Read the model definition and answer for the solid it produces. Units are mm, in the model's axes. Face numbers are marked on the shaded views. Coordinates: 2 decimals unless noted, no trailing zeros. Order: outer loops, then holes, each group sorted by start corner. A loop starts at its lowest first (then second) coordinate and runs counter-clockwise, first axis right, second up. Notation, with made-up numbers: M 80.5,45.25 L 97.5,45.25 A24 ccw 97.5,74.25 Z; hole C 80.25,78 d6. An arc over 180 degrees is marked long. One line per question, with ' | ' between items. Start each with the question number.
1) Consider probe 1 along Z at (x, y) = (-8, 16.5); probe 2 along X at (y, z) = (7, -41) (3 decimals); probe 3 along Y at (x, z) = (0, -50.95). Determine where each line is inside the solid, lowest interval first.
2) Find section A-A, the plane x = 0. Count the separate pieces of the cut face and the enclosed holes in it, plus the area to 3 significant figures.
3) Find section B-B, the plane y = 13. Write down the section's boundary in (x, z) (3 decimals).
4) The mould has two halves that part along Z. Classify the marked faces 1 and 2: +Z half, -Z half, draft (parallel to the pull), parting line (faces both ways), or undercut.
5) Find section C-C, the plane z = -32.5. Write down the section's boundary in (x, y) (3 decimals), plus the area to 3 significant figures.
6) Given P1, Ø8, axis at y = 6.5, z = 22.5, coming from the +X side (3 decimals); P2, Ø5, axis at y = 8.5, z = -14.5, coming from the -X side (3 decimals); P3, Ø10, axis at x = 0.5, y = 11.5, coming from the +Z side; P4, Ø9, axis at x = 0, y = 11.43, coming from the -Z side, each flat-ended and moving along its own axis, determine where each tip first touches the part or whether it passes through.
Autodesk Inventor part; units mm, degrees
ref_plane "YZ Plane" through (0, 0, 0) normal (1, 0, 0) x (0, 1, 0)
ref_plane "XZ Plane" through (0, 0, 0) normal (0, 1, 0) x (-1, 0, 0)
ref_plane "XY Plane" through (0, 0, 0) normal (0, 0, 1) x (1, 0, 0)
sketch "Sketch1" plane through (0, 0, 0) normal (0, 1, 0) x (-1, 0, 0)
  line L0 (-6.985, 50) -> (6.985, 50)
  line L1 (6.985, 50) -> (6.985, -50)
  line L2 (6.985, -50) -> (-6.985, -50)
  line L3 (-6.985, -50) -> (-6.985, 50)
  line L4 (-6.985, 50) -> (6.985, -50) construction
  line L5 (6.985, 50) -> (-6.985, -50) construction
  point P0 (0, 0)
  dimension "d0" = 13.97
  dimension "d1" = 100
extrude "Extrusion1" add sketch "Sketch1" along normal blind 2
sketch "Sketch2" plane through (0, 0, 0) normal (0, -1, 0) x (1, 0, 0)
  point P0 (0, 0)
sketch "Sketch3" plane through (0, 2, 0) normal (0, 1, 0) x (1, 0, 0)
  point P0 (0, 0)
sketch "Sketch4" plane through (0, 0, 0) normal (0, -1, 0) x (1, 0, 0)
  line L0 (6.985, -50) -> (-6.985, -50)
  line L1 (-6.985, -50) -> (-9.485, -50)
  line L2 (-9.485, -50) -> (-9.485, 50)
  line L3 (-9.485, 50) -> (-6.985, 50)
  line L4 (-6.985, 50) -> (-6.985, -50)
  line L5 (-6.985, 50) -> (6.985, 50)
  line L6 (6.985, 50) -> (9.485, 50)
  line L7 (9.485, 50) -> (9.485, -50)
  line L8 (9.485, -50) -> (6.985, -50)
  line L9 (6.985, -50) -> (6.985, 50)
  point P0 (0, 0)
  dimension "d4" = 2.5
  dimension "d5" = 2.5
extrude "Extrusion2" add sketch "Sketch4" against normal blind 10.89 contours L9 L6 L7 L8 | L1 L2 L3 L4
sketch "Sketch5" plane through (0, 10.89, 0) normal (0, 1, 0) x (1, 0, 0)
  line L0 (9.485, 50) -> (9.485, -50)
  line L1 (6.985, 50) -> (-6.985, 50)
  line L2 (9.485, -50) -> (6.985, -50)
  line L3 (6.985, -50) -> (6.985, 50)
  line L4 (6.985, 50) -> (9.485, 50)
  line L5 (9.485, 50) -> (9.485, -50)
  point P0 (0, 0)
extrude "Extrusion3" cut sketch "Sketch5" against normal blind 3.14
sketch "Sketch6" plane through (0, 10.89, 0) normal (0, 1, 0) x (1, 0, 0)
  line L0 (-6.985, 50) -> (-6.985, -50)
  line L1 (-9.485, -50) -> (-9.485, 50)
  line L2 (-6.985, -50) -> (-9.485, -50)
  line L3 (-9.485, -50) -> (-9.485, 50)
  line L4 (-9.485, 50) -> (-6.985, 50)
  line L5 (-6.985, 50) -> (-6.985, -50)
  point P0 (0, 0)
extrude "Extrusion4" cut sketch "Sketch6" against normal blind 2.14
sketch "Sketch7" plane through (0, 8.75, 0) normal (0, 1, 0) x (1, 0, 0)
  line L0 (-6.985, 50) -> (-6.985, -50)
  line L1 (-9.485, -50) -> (-9.485, 50)
  line L2 (-6.985, 0) -> (-9.485, 0)
  line L3 (-9.485, 0) -> (-9.485, 3.5)
  line L4 (-9.485, 3.5) -> (-6.985, 3.5)
  line L5 (-6.985, 3.5) -> (-6.985, 0)
  point P0 (0, 0)
  dimension "d12" = 3.5
extrude "Extrusion5" add sketch "Sketch7" along normal blind 2.14
fillet "Fillet1" radius 7 2 edges at (-8.235, 8.75, -3.5) (-8.235, 10.89, -3.5)
sketch "Sketch8" plane through (-9.485, 0, 50) normal (0, 0, 1) x (1, 0, 0)
  line L0 (0, 0) -> (0, 8.75) construction
  line L1 (0, 0) -> (18.97, 0) construction
  line L2 (18.97, 0) -> (18.97, 11.43) construction
  line L3 (18.97, 11.43) -> (0, 11.43) construction
  line L4 (0, 11.43) -> (0, 0) construction
  line L5 (0, 0) -> (18.97, 0)
  line L6 (18.97, 0) -> (18.97, 22.5)
  line L7 (18.97, 22.5) -> (0, 22.5)
  line L8 (0, 22.5) -> (0, 0)
  circle A0 centre (9.485, 11.43) radius 7.9875
  point P0 (9.485, 0)
  dimension "d16" = 11.43
  dimension "d17" = 22.5
  dimension "d18" = 15.975
extrude "Extrusion6" add sketch "Sketch8" along normal blind 7
sketch "Sketch9" plane through (9.485, 0, -50) normal (0, 0, -1) x (-1, 0, 0)
  line L0 (0, 22.5) -> (18.97, 22.5)
  line L1 (0, 0) -> (18.97, 0)
  line L2 (18.97, 0) -> (18.97, 22.5)
  line L3 (18.97, 22.5) -> (0, 22.5)
  line L4 (0, 22.5) -> (0, 0)
  circle A0 centre (9.485, 11.43) radius 7.9875
  circle A1 centre (9.485, 11.43) radius 7.9875
  point P0 (9.485, 0)
extrude "Extrusion7" add sketch "Sketch9" along normal blind 7
fillet "Fillet2" radius 5 4 edges at (-9.485, 22.5, -53.5) (9.485, 22.5, 53.5) (-9.485, 22.5, 53.5) (9.485, 22.5, -53.5)
sketch "Sketch10" plane through (-9.485, 0, 50) normal (0, 0, -1) x (-1, 0, 0)
  circle A0 centre (-9.485, 11.43) radius 7.9875
  circle A1 centre (-9.485, 11.43) radius 7.9875
  circle A2 centre (-9.485, 11.43) radius 3.175 construction
  circle A3 centre (-9.485, 11.43) radius 5
  point P0 (-9.485, 0)
  dimension "d24" = 6.35
  dimension "d25" = 10
extrude "Extrusion8" add sketch "Sketch10" against normal blind 2
sketch "Sketch11" plane through (9.485, 0, -50) normal (0, 0, 1) x (1, 0, 0)
  circle A0 centre (-9.485, 11.43) radius 5
  circle A1 centre (-9.485, 11.43) radius 7.9875
  circle A2 centre (-9.485, 11.43) radius 5
  point P0 (-9.485, 0)
  dimension "d28" = 10
extrude "Extrusion9" add sketch "Sketch11" against normal blind 2
sketch "Sketch12" plane through (0, 8.75, 0) normal (0, 1, 0) x (1, 0, 0)
  point P0 (0, 0)
sketch "Sketch13" plane through (0, 2, 0) normal (0, 1, 0) x (1, 0, 0)
  line L0 (6.985, 50) -> (-6.985, 50) construction
  line L1 (-6.985, 50) -> (-6.985, 8.5379) construction
  line L2 (6.985, 50) -> (-6.985, 50) construction
  line L3 (-6.985, 50) -> (-6.985, 36.03) construction
  line L4 (-6.985, 36.03) -> (6.985, 36.03) construction
  line L5 (6.985, 36.03) -> (6.985, 50) construction
  circle A0 centre (0, 43.015) radius 1.5875
  point P0 (0, 0)
  dimension "d31" = 13.97
  dimension "d32" = 3.175
extrude "Extrusion10" cut sketch "Sketch13" against normal blind 2
fillet "Fillet3" radius 2 1 edges at (-1.5875, 2, -43.015)
sketch "Sketch14" plane through (0, 2, 0) normal (0, 1, 0) x (1, 0, 0)
  circle A0 centre (0, 43.015) radius 1.5875 construction
  line L0 (0, 43.015) -> (-9.485, 43.015) construction
  line L1 (-9.485, 8.5379) -> (-9.485, 50) construction
  line L2 (0, 43.015) -> (0, 50) construction
  line L3 (6.985, 50) -> (-6.985, 50) construction
  point P0 (0, 0)
  dimension "d36" = 6.985
  dimension "d37" = 9.485
sketch "Sketch15" plane through (-9.485, 8.75, 0) normal (-1, 0, 0) x (0, 0, 1)
  point P0 (0, -8.75)
sketch "Sketch16" plane through (9.485, 0, 57) normal (1, 0, 0) x (0, 0, -1)
  line L0 (107, 7.75) -> (7, 7.75) construction
  line L1 (114, 0) -> (0, 0) construction
  line L2 (7, 7.75) -> (14.75, 7.75) construction
  line L3 (14.75, 7.75) -> (14.75, 0) construction
  line L4 (14.75, 0) -> (7, 0) construction
  line L5 (7, 0) -> (7, 7.75) construction
  line L6 (13.625, 1.125) -> (8.125, 1.125)
  line L7 (8.125, 1.125) -> (8.125, 6.625)
  line L8 (8.125, 6.625) -> (13.625, 6.625)
  line L9 (13.625, 6.625) -> (13.625, 1.125)
  line L10 (13.625, 1.125) -> (8.125, 6.625) construction
  line L11 (8.125, 1.125) -> (13.625, 6.625) construction
  circle A0 centre (10.875, 3.875) radius 2
  point P0 (57, 0)
  dimension "d38" = 7.75
  dimension "d39" = 5.5
  dimension "d40" = 5.5
  dimension "d41" = 4
extrude "Extrusion11" add sketch "Sketch16" along normal blind 2.5
sketch "Sketch17" plane through (9.485, 3.875, 46.125) normal (1, 0, 0) x (0, 0, -1)
  circle A0 centre (0, 0) radius 2 construction
  line L0 (0, 0) -> (-3.875, 0) construction
  line L1 (-3.875, 0) -> (-3.875, -3.875) construction
  line L2 (-3.875, -3.875) -> (0, -3.875) construction
  line L3 (0, -3.875) -> (0, 0) construction
  point P0 (46.125, -3.875)
  dimension "d44" = 3.875
  dimension "d45" = 3.875
sketch "Sketch18" plane through (0, 0, 0) normal (0, -1, 0) x (1, 0, 0)
  point P0 (0, 0)
sketch "Sketch19" plane through (-9.485, 8.75, 0) normal (-1, 0, 0) x (0, 0, 1)
  point P0 (0, -8.75)
sketch "Sketch20" plane through (-9.485, 8.75, 0) normal (-1, 0, 0) x (0, 0, 1)
  line L0 (50, -2.32) -> (50, 7.68) construction
  line L1 (-57, -8.75) -> (57, -8.75) construction
  line L2 (50, 0) -> (41.25, 0) construction
  line L3 (41.25, 0) -> (41.25, -8.75) construction
  line L4 (41.25, -8.75) -> (50, -8.75) construction
  line L5 (50, -8.75) -> (50, 0) construction
  circle A0 centre (45.625, -4.375) radius 1.5 construction
  circle A1 centre (45.625, -4.375) radius 1.5
  point P0 (0, -8.75)
  dimension "d46" = 8.75
  dimension "d47" = 3
extrude "Extrusion12" add sketch "Sketch20" along normal blind 3
sketch "Sketch21" plane through (-9.485, 8.75, 0) normal (-1, 0, 0) x (0, 0, 1)
  circle A0 centre (45.625, -4.375) radius 1.5 construction
  line L0 (45.625, -4.375) -> (50, -4.375) construction
  line L1 (57, -8.75) -> (-57, -8.75) construction
  line L2 (45.625, -4.375) -> (50, -4.375) construction
  line L3 (50, -4.375) -> (50, -8.75) construction
  line L4 (50, -8.75) -> (45.625, -8.75) construction
  line L5 (45.625, -8.75) -> (45.625, -4.375) construction
  point P0 (0, -8.75)
  point P1 (50, 0)
  dimension "d50" = 4.375
  dimension "d51" = 4.375
properties part number "mtv_frontAxelHolder(4_30)"
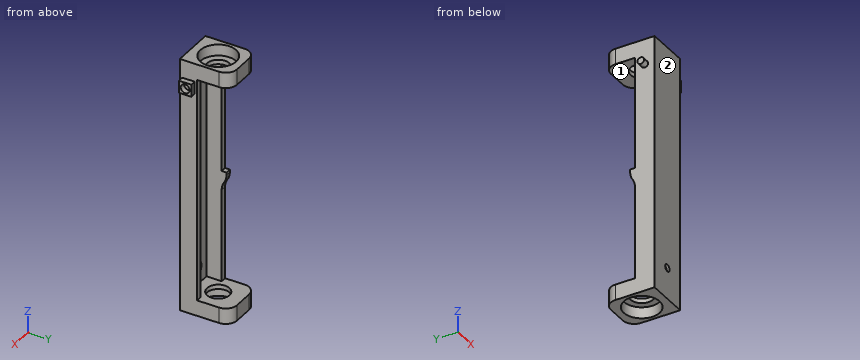
Report:
1) probe 1: z = -57 to -50, 50 to 57 | probe 2: x = -9.485 to -6.985, 6.985 to 9.485 | probe 3: y = 0 to 6.43, 16.43 to 22.5
2) separate pieces: 4 | enclosed holes: 0 | area: 307 mm^2
3) outline: M -9.485,-57 L -7.832,-57 L -7.832,-52 L -4.747,-52 L -4.747,-50 L -9.485,-50 Z; M -9.485,50 L -4.747,50 L -4.747,52 L -7.832,52 L -7.832,57 L -9.485,57 Z; M 4.747,-52 L 7.832,-52 L 7.832,-57 L 9.485,-57 L 9.485,-50 L 4.747,-50 Z; M 4.747,50 L 9.485,50 L 9.485,57 L 7.832,57 L 7.832,52 L 4.747,52 Z
4) face 1: undercut | face 2: draft
5) outline: M -9.485,0 L 9.485,0 L 9.485,7.75 L 6.985,7.75 L 6.985,2 L -6.985,2 L -6.985,8.75 L -9.485,8.75 Z | area: 69.2 mm^2
6) P1: stops at x = 9.485 | P2: stops at x = -9.485 | P3: stops at z = 52 | P4: passes through
